Source: CAD feature listing. Evaluate the final solid. Frame: model axes, mm. A direction names the side the tool comes from. Round coordinates to 2 decimals unless told otherwise and drop trailing zeros. Loops run counter-clockwise (first coordinate to the right, second up) from the corner with the lowest first, then second, coordinate; pieces in that order, holes last. Notation, with made-up numbers: (-20, -1) - (37, -1) arc R21 cw to (37, 33) - close; hole circle Ø1 at (57.25, 57). An arc over 180 degrees is marked (long way). Use CSV: the item, a comma, the result in double quotes. Start each with the question number.
from build123d import *

# Parameters (mm, degrees)
SKETCH1_R           = 1.6
SKETCH1_W           = 21
SKETCH1_H           = 41
BOSS_EXTRUDE1_DEPTH = 11
SKETCH6_W           = 21
SKETCH6_H           = 0.1
CUT_EXTRUDE1_DEPTH  = 91.428148273
SKETCH7_W           = 21
SKETCH7_H           = 41.2
SKETCH7_R           = 1.6
CUT_EXTRUDE2_DEPTH  = 11


with BuildPart() as part:
    # Sketch1 → Boss-Extrude1 (new body)
    with BuildSketch(Plane.XY):
        with BuildLine():
            Line((-20, 70), (-20, -50))
            ThreePointArc((-20, -50), (-2.5, -67.5), (15, -50))
            Line((15, -50), (15, 70))
            ThreePointArc((15, 70), (-2.5, 87.5), (-20, 70))
        make_face()
        with Locations((-7.5, 79.5)):
            Circle(SKETCH1_R, mode=Mode.SUBTRACT)
        with Locations(Location((2.5, 79.5, 0), (0, 0, 180))):
            Circle(SKETCH1_R, mode=Mode.SUBTRACT)
        with Locations((2.5, 30.5)):
            Circle(SKETCH1_R, mode=Mode.SUBTRACT)
        with Locations(Location((-7.5, 30.5, 0), (0, 0, 180))):
            Circle(SKETCH1_R, mode=Mode.SUBTRACT)
        with Locations((-2.5, 55)):
            Rectangle(SKETCH1_W, SKETCH1_H, mode=Mode.SUBTRACT)
    extrude(amount=BOSS_EXTRUDE1_DEPTH)

    # Sketch6 → Cut-Extrude1 (cut, through all)
    with BuildSketch(Plane.XY.offset(11)):
        with Locations((-2.5, 75.55)):
            Rectangle(SKETCH6_W, SKETCH6_H)
        with Locations((-2.5, 34.45)):
            Rectangle(SKETCH6_W, SKETCH6_H)
    extrude(amount=-CUT_EXTRUDE1_DEPTH, mode=Mode.SUBTRACT)

    # Sketch7 → Cut-Extrude2 (cut)
    with BuildSketch(Plane(origin=(0, 0, 0), x_dir=(-1, 0, 0), z_dir=(0, 0, -1))):
        with Locations((2.5, -35)):
            Rectangle(SKETCH7_W, SKETCH7_H)
        with Locations((-2.5, -10.5)):
            Circle(SKETCH7_R)
        with Locations((7.5, -10.5)):
            Circle(SKETCH7_R)
        with Locations((-2.5, -59.5)):
            Circle(SKETCH7_R)
        with Locations((7.5, -59.5)):
            Circle(SKETCH7_R)
    extrude(amount=-CUT_EXTRUDE2_DEPTH, mode=Mode.SUBTRACT)


solid = part.part
1. Section query B-B on y = -10.5. Return the cut outline in (x, z).
2. Section query A-A on x = -2.5. Return the cut outline in (y, z), and give its area (3 significant figures).
3. Reachability of faces 1 (the flat face through (-13, -35, 5)), 2 (the flat face through (-3, 11, 0)) from +Z, -Z, +X, -X, +Y, -Y: full face, straight path, thin tool, end or side. Return the list, or none.
4. Section query D-D on y = -40. Return the cut outline in (x, z), and give its area (3 significant figures).
5. Section query C-C on z = 5.25. Give the number of separate pieces and of enclosed holes in the cut face, and give its area (3 significant figures).
6. Line query: line 1 along X through (y, z) = (53, 10); line 2 along X through (y, z) = (79.5, 3); line 3 along Y through (x, z) = (-9.5, 7.5). Output: solid intervals per line, ascending.
7. Contact query for flat-ended pins moving along their axis: P1, Ø2.5, axis at x = 2.5, y = 79.5, coming from the +Z side; P2, Ø5, axis at x = -13, z = 1, coming from the +Y side; P3, Ø1.5, axis at x = 9, z = 6, coming from the +Y side; P4, Ø3.5, axis at x = -5.5, z = 6, coming from the +Y side. Output: stop coordinate, or through.
8. Mould query, pull axis Y, two halves, no side actions, for faces 3 (the cylindrical face through (-2.115, 87.496, 5.423)), 4 (the flat face through (15, 9, 5)), 5 (the cylindrical face through (-7.292, -57.914, 5.423)). Classes: +Y half, -Y half, draft (parallel to the pull), parting line (faces both ways), or undercut.
Values:
1,outline,"(-20, 0) - (-9.1, 0) - (-9.1, 11) - (-20, 11) - close; (-5.9, 0) - (0.9, 0) - (0.9, 11) - (-5.9, 11) - close; (4.1, 0) - (15, 0) - (15, 11) - (4.1, 11) - close"
2,outline,"(-67.5, 0) - (-55.6, 0) - (-55.6, 11) - (-67.5, 11) - close; (-14.4, 0) - (34.4, 0) - (34.4, 11) - (-14.4, 11) - close; (75.6, 0) - (87.5, 0) - (87.5, 11) - (75.6, 11) - close"
2,area,"799 mm^2"
3,face 1,"+Z, -Z"
3,face 2,"-Z, +X, -X, +Y, -Y"
4,outline,"(-20, 0) - (-13, 0) - (-13, 11) - (-20, 11) - close; (8, 0) - (15, 0) - (15, 11) - (8, 11) - close"
4,area,"154 mm^2"
5,separate pieces,"1"
5,enclosed holes,"10"
5,area,"3,370 mm^2"
6,line 1,"x = -20 to -13, 8 to 15"
6,line 2,"x = -17.2 to -9.1, -5.9 to 0.9, 4.1 to 12.2"
6,line 3,"y = -66.04 to -55.6, -14.4 to 34.4, 75.6 to 86.04"
7,P1,"passes through"
7,P2,"stops at y = 85.56"
7,P3,"stops at y = 83.81"
7,P4,"stops at y = 87.46"
8,face 3,"+Y half"
8,face 4,"draft"
8,face 5,"undercut"
